Verification items for the finished model (mm, model axes). Give positions to 0.01 mm unless a question says otherwise; leave off trailing zeros. Order: outer loops, then holes, each group sorted by start corner. A loop starts at its lowest first (then second) coordinate and runs counter-clockwise, first axis right, second up.
from build123d import *

# Parameters (mm, degrees)
F0_W     = 1219.2
F0_H     = 127
F1_DEPTH = 101.6
F3_DEPTH = 1219.2


with BuildPart() as f1:
    # F0 (on Top) → F1 (new body)
    with BuildSketch(Plane.XY):
        with Locations((609.6, 63.5)):
            Rectangle(F0_W, F0_H)
    extrude(amount=F1_DEPTH)

    # F2 (on face) → F3 (cut, through all)
    with BuildSketch(Plane.YZ.offset(1219.2)):
        with BuildLine():
            Line((9.579805, 101.6), (0, 101.6))
            Line((0, 101.6), (0, 0))
            Line((0, 0), (7.050204, 0))
            Line((7.050204, 0), (14.157143, 0))
            ThreePointArc((14.157143, 0), (4.627971, 4.21213), (1.328974, 14.094627))
            Line((1.328974, 14.094627), (8.66489, 91.896731))
            ThreePointArc((8.66489, 91.896731), (12.118215, 98.810986), (19.326112, 101.6))
            Line((19.326112, 101.6), (9.579805, 101.6))
        make_face()
        with BuildLine():
            Line((117.420195, 101.6), (107.673888, 101.6))
            ThreePointArc((107.673888, 101.6), (114.881785, 98.810986), (118.33511, 91.896731))
            Line((118.33511, 91.896731), (125.671026, 14.094627))
            ThreePointArc((125.671026, 14.094627), (122.372029, 4.21213), (112.842857, 0))
            Line((112.842857, 0), (119.949796, 0))
            Line((119.949796, 0), (127, 0))
            Line((127, 0), (127, 101.6))
            Line((127, 101.6), (117.420195, 101.6))
        make_face()
    extrude(amount=-F3_DEPTH, mode=Mode.SUBTRACT)


solid = f1.part
(1) Section check B-B, the plane z = 31.5. Enter the section's corners in (x, y), then the cut area to 3 significant figures.
Solved:
outline: (0, 2.97) - (1219.2, 2.97) - (1219.2, 124.03) - (0, 124.03) - close
area: 148,000 mm2
(2) Scan lines: line 1 (Z direction, x = 1158.5, y = 18.5); line 2 (Y direction, x = 1019, z = 14); line 3 (Y direction, x = 994, z = 16.5). Record each from-to range of solid material in increasing order.
Solved:
line 1: z = 0 to 101.57
line 2: y = 1.32 to 125.68
line 3: y = 1.56 to 125.44
(3) Go/stop test with a flat-tipped pin: pin 1 (10 mm diameter, centred on x = 591.5, z = 35, fed in from +Y). Record where the tip stops, or that it passes through.
Solved:
pin 1: stops at y = 124.17
(4) Section check A-A, the plane x = 1142. Enter the section's corners in (y, z).
Solved:
outline: (1.33, 14.09) arc R12.89 ccw to (14.16, 0) - (112.84, 0) arc R12.89 ccw to (125.67, 14.09) - (118.34, 91.9) arc R10.71 ccw to (107.67, 101.6) - (19.33, 101.6) arc R10.71 ccw to (8.66, 91.9) - close
